```python
from build123d import *

# Parameters (mm, degrees)
EXTRUDE_1_DEPTH = 5
EXTRUDE_2_DEPTH = 5


with BuildPart() as part:
    # 草图1 → 凸台-拉伸1 (new body)
    with BuildSketch(Plane(origin=(0, 0, 0), x_dir=(1, 0, 0), z_dir=(0, 1, 0))):
        with BuildLine():
            Line((-32, 0), (-30, 0))
            ThreePointArc((-30, 0), (0, 30), (30, 0))
            Line((30, 0), (32, 0))
            ThreePointArc((32, 0), (0, 32), (-32, 0))
        make_face()
    extrude(amount=EXTRUDE_1_DEPTH)

    # 草图2 → 凸台-拉伸2 (add)
    with BuildSketch(Plane(origin=(0, 0, 0), x_dir=(1, 0, 0), z_dir=(0, 1, 0))):
        Polygon((5, 37), (0, 37), (-5, 37), (-5, 30.465276436), (5, 30.465276436), align=None)
    extrude(amount=EXTRUDE_2_DEPTH)


solid = part.part
```
Verification items for the finished model (mm, model axes). A direction names the side the tool comes from. Round coordinates to 2 decimals unless told otherwise and drop trailing zeros. Order: outer loops, then holes, each group sorted by start corner. A loop starts at its lowest first (then second) coordinate and runs counter-clockwise, first axis right, second up. Notation, with made-up numbers: (10.25, 35) - (32.25, 35) arc R27 ccw to (32.25, 56) - close; hole circle Ø6 at (89.25, 66). An arc over 180 degrees is marked (long way). Use CSV: the item, a comma, the result in double quotes. Start each with the question number.
1) Section check B-B, the plane z = -16.5. Record the cut outline in (x, y), plus the area to 3 significant figures.
2) Mould release check, pull along X, two halves, no side actions. Record for faces 1 (the flat face through (0, 2, -37)), 2 (the flat face through (5, 2, -34)), 3 (the cylindrical face through (-24.124, 2.465, -21.024)), 4 (the cylindrical face through (-0.66, 2.465, -29.993)): +X half, -X half, draft (parallel to the pull), parting line (faces both ways), or undercut.
3) Go/stop test with flat-tipped pins: P1, Ø1.5, axis at y = 2.5, z = -35, coming from the -X side; P2, Ø2.5, axis at y = 3, z = -33.5, coming from the +X side; P3, Ø1, axis at y = 3, z = -20.5, coming from the +X side. Record where each tip stops, or that it passes through.
4) Thickness scan on L1, parallel to X at y = 0.6, z = -33.5; L2, parallel to X at y = 1.95, z = -4; L3, parallel to X at y = 1.95, z = -21. Record the ranges inside material, lowest first.
5) Section check D-D, the plane x = 0. Record the cut outline in (y, z), plus the area to 3 significant figures.
6) Access from +Z, -Z, +X, -X, +Y, -Y to the whole of each face (thin tool, end or side, straight path). Record for faces 5 (the flat face through (31, 2, 0)), 6 (the flat face through (-5, 2, -34)).
7) Section check C-C, the plane x = 6.5. Record the cut outline in (y, z), plus the area to 3 significant figures.
8) Section check A-A, the plane y = 3.2. Record the cut outline in (x, z).
Answers:
1,outline,"(-27.42, 0) - (-25.05, 0) - (-25.05, 5) - (-27.42, 5) - close; (25.05, 0) - (27.42, 0) - (27.42, 5) - (25.05, 5) - close"
1,area,"23.6 mm²"
2,face 1,"draft"
2,face 2,"+X half"
2,face 3,"-X half"
2,face 4,"undercut"
3,P1,"stops at x = -5"
3,P2,"stops at x = 5"
3,P3,"stops at x = 24.98"
4,L1,"x = -5 to 5"
4,L2,"x = -31.75 to -29.73, 29.73 to 31.75"
4,L3,"x = -24.15 to -21.42, 21.42 to 24.15"
5,outline,"(0, -37) - (5, -37) - (5, -30) - (0, -30) - close"
5,area,"35.0 mm²"
6,face 5,"+Z, +X, -X, +Y, -Y"
6,face 6,"-Z, -X, +Y, -Y"
7,outline,"(0, -31.33) - (5, -31.33) - (5, -29.29) - (0, -29.29) - close"
7,area,"10.2 mm²"
8,outline,"(-32, 0) arc R32 ccw to (-5, -31.61) - (-5, -37) - (5, -37) - (5, -31.61) arc R32 ccw to (32, 0) - (30, 0) arc R30 cw to (-30, 0) - close"
